```python
from build123d import *

# Parameters (mm, degrees)
SKETCH2_W          = 52.291467072
SKETCH2_H          = 20.32
BASE_FLANGE1_DEPTH = 3.175
EDGE_FLANGE1_DEPTH = 52.291467072


# Sheet-metal steps are written as plain solids
with BuildPart() as part:
    # Sketch2 → Base-Flange1 (new body)
    with BuildSketch(Plane.XY):
        with Locations((26.145733536, 10.16)):
            Rectangle(SKETCH2_W, SKETCH2_H)
    extrude(amount=-BASE_FLANGE1_DEPTH)

    # Edge-Flange1 section (across the edge) → Edge-Flange1 (add)
    with BuildSketch(Plane(origin=(52.291467072, 23.495, 0), x_dir=(0, -1, 0), z_dir=(-1, 0, 0))):
        with BuildLine():
            Line((-3.175, 3.175), (-3.175, 17.145))
            Line((-3.175, 17.145), (0, 17.145))
            Line((0, 17.145), (0, 3.175))
            ThreePointArc((0, 3.175), (0.92993597, 0.92993597), (3.175, 0))
            Line((3.175, 0), (3.175, -3.175))
            ThreePointArc((3.175, -3.175), (-1.315128061, -1.315128061), (-3.175, 3.175))
        make_face()
    extrude(amount=EDGE_FLANGE1_DEPTH)


solid = part.part
```
Read the model definition and answer for the solid it produces. Units are mm, in the model's axes. A direction names the side the tool comes from. Give positions to 0.01 mm unless a question says otherwise; leave off trailing zeros. Write each loop counter-clockwise with the first axis right and the second up, starting at its lowest first coordinate (ties: lowest second). Pieces come first, ordered by that corner, then holes. Notation, with made-up numbers: (-25.75, 77.5) - (2.25, 77.5) arc R26 cw to (2.25, 93.5) - close; hole circle Ø10 at (-17.5, 53). An arc over 180 degrees is marked (long way). Write item = value, one per line. Start each with the question number.
Item 1: Find section B-B (y = 19). Give the vertices of the cut face in (x, z) (3 decimals).
Item 2: Find the intervals of material crossed by probe 1 along Z at (x, y) = (32, 4.5) (3 decimals); probe 2 along Y at (x, z) = (31.5, 14.75) (3 decimals); probe 3 along Z at (x, y) = (18, 24.75) (3 decimals), in increasing order. Write a range as [from, to].
Item 3: Each of these flat-tipped pins is pushed along its axis until it touches: P1, Ø4, axis at x = 37.5, z = 9, coming from the -Y side (3 decimals); P2, Ø8, axis at x = 36, y = 7.5, coming from the +Z side; P3, Ø4, axis at x = 23.5, z = 4.5, coming from the -Y side. Where does it stop, or does it pass through?
Item 4: Find section A-A (x = 7.5). Give the vertices of the cut face in (y, z) (3 decimals), then the cut area to 3 significant figures.
Item 5: A tool of negligible diameter and unlimited length cuts with its end or side. For faces 1 (the flat face through (26, 10, 0)), 2 (the flat face through (26, 10, -3.175)), from which of +Z, -Z, +X, -X, +Y, -Y can it reach the whole face along a straight path? Write none if from no direction.
Item 6: Find section C-C (z = 12.5). Give the vertices of the cut face in (x, y) (3 decimals).
Response:
q1.outline = (0, -3.175) - (52.291, -3.175) - (52.291, 0) - (0, 0) - close
q2.probe_1 = [-3.175, 0]
q2.probe_2 = [23.495, 26.67]
q2.probe_3 = [-1.374, 17.145]
q3.P1 = 23.495
q3.P2 = 0
q3.P3 = 23.42
q4.outline = (0, -3.175) - (20.32, -3.175) arc R6.35 ccw to (26.67, 3.175) - (26.67, 17.145) - (23.495, 17.145) - (23.495, 3.175) arc R3.175 cw to (20.32, 0) - (0, 0) - close
q4.area = 133 mm²
q5.face_1 = +Z, +X, -X, -Y
q5.face_2 = -Z, +X, -X, +Y, -Y
q6.outline = (0, 23.495) - (52.291, 23.495) - (52.291, 26.67) - (0, 26.67) - close
